from build123d import *

# Parameters (mm, degrees)
ESBO_O1_W                = 113
ESBO_O1_H                = 26.5
RESSALTO_EXTRUS_O1_DEPTH = 5
ESBO_O2_W                = 5
ESBO_O2_H                = 7.62
CORTE_EXTRUS_O1_DEPTH    = 5
CORTE_EXTRUS_O2_DEPTH    = 5
ESBO_O4_R                = 1.6
CORTE_EXTRUS_O3_DEPTH    = 10


with BuildPart() as part:
    # Esboço1 → Ressalto-extrusão1 (new body)
    with BuildSketch(Plane(origin=(0, 0, 0), x_dir=(1, 0, 0), z_dir=(0, 1, 0))):
        with Locations((-20.23644711, -18.909257917)):
            Rectangle(ESBO_O1_W, ESBO_O1_H)
    extrude(amount=RESSALTO_EXTRUS_O1_DEPTH)

    # Esboço2 → Corte-extrusão1 (cut)
    with BuildSketch(Plane(origin=(0, 5, 0), x_dir=(1, 0, 0), z_dir=(0, 1, 0))):
        with Locations((13.76355289, -18.914257917)):
            Rectangle(ESBO_O2_W, ESBO_O2_H)
        with Locations((-54.23644711, -18.914257917)):
            Rectangle(ESBO_O2_W, ESBO_O2_H)
    extrude(amount=-CORTE_EXTRUS_O1_DEPTH, mode=Mode.SUBTRACT)

    # Esboço3 → Corte-extrusão2 (cut)
    with BuildSketch(Plane(origin=(0, 5, 0), x_dir=(1, 0, 0), z_dir=(0, 1, 0))):
        Polygon((-76.73644711, -17.909257917), (-73.23644711, -17.909257917), (-73.23644711, -16.109257917), (-71.73644711, -16.109257917), (-71.73644711, -17.909257917), (-69.73644711, -17.909257917), (-69.73644711, -19.909257917), (-71.73644711, -19.909257917), (-71.73644711, -21.709257917), (-73.23644711, -21.709257917), (-73.23644711, -19.909257917), (-76.73644711, -19.909257917), align=None)
        Polygon((-51.73644711, -17.909257917), (-48.23644711, -17.909257917), (-48.23644711, -16.109257917), (-46.73644711, -16.109257917), (-46.73644711, -17.909257917), (-44.73644711, -17.909257917), (-44.73644711, -19.909257917), (-46.73644711, -19.909257917), (-46.73644711, -21.709257917), (-48.23644711, -21.709257917), (-48.23644711, -19.909257917), (-51.73644711, -19.909257917), align=None)
    corte_extrus_o2 = extrude(amount=-CORTE_EXTRUS_O2_DEPTH, mode=Mode.SUBTRACT)

    # Espelhar1: Corte-extrusão2 across plane
    add(corte_extrus_o2.mirror(Plane.ZY.offset(20.23644711)), mode=Mode.SUBTRACT)

    # Esboço4 → Corte-extrusão3 (cut)
    with BuildSketch(Plane(origin=(0, 0, 0), x_dir=(-1, 0, 0), z_dir=(0, -1, 0))):
        with Locations(Location((1.56644711, -10.659257917, 0), (0, 0, 90))):
            Circle(ESBO_O4_R)
        with Locations(Location((38.90644711, -10.659257917, 0), (0, 0, 90))):
            Circle(ESBO_O4_R)
    extrude(amount=-CORTE_EXTRUS_O3_DEPTH, mode=Mode.SUBTRACT)


solid = part.part
Part model, mm, in its own coordinate system. A direction names the side the tool comes from. Coordinates: 2 decimals unless noted, no trailing zeros. Loops run counter-clockwise (first coordinate to the right, second up) from the corner with the lowest first, then second, coordinate; pieces in that order, holes last. Notation, with made-up numbers: (43, 62.5) - (88, 62.5) arc R35 ccw to (88, 97.5) - close; hole circle Ø10 at (75, -30). An arc over 180 degrees is marked (long way). Write each question's results on one line, items separated by ' | '. Start each with the question number.
Q1. Which spindle directions (+Z, -Z, +X, -X, +Y, -Y) get a long thin tool onto all of the face, cutting with end or side? Do faces 1 (the flat face through (-75, 3, 17.909)), 2 (the flat face through (34, 3, 19.909)), 3 (the flat face through (-51.736, 3, 17)). Say none if no direction does.
Q2. Two-plate mould, pull along Z, no slides. Class faces 4 (the flat face through (-76.736, 2, 26)), 5 (the flat face through (31.264, 3, 17)): +Z half, -Z half, draft (parallel to the pull), parting line (faces both ways), or undercut.
Q3. Drop a flat-ended pin along its axis: pin 1 Ø1.9 at (x, z) = (-38.91, 10.66) entering from +Y. Give the stop position or say it passes through.
Q4. Probe line 1 along X through (y, z) = (3.5, 18); line 2 along Z through (x, y) = (13.5, 2.8); line 3 along Z through (x, y) = (-48, 3.45). List the from-to ranges inside material, lowest first.
Q5. Slice it at A-A on x = 13. Give the cut face in (y, z).
Q6. Slice it at B-B on y = 3.55. Give the number of separate pieces and of enclosed holes in the cut face, and give its area (3 significant figures).
Answer:
1) face 1: -X, +Y, -Y | face 2: +X, +Y, -Y | face 3: +Y, -Y
2) face 4: draft | face 5: undercut
3) pin 1: passes through
4) line 1: x = -69.74 to -56.74, -44.74 to 4.26, 16.26 to 29.26 | line 2: z = 5.66 to 15.1, 22.72 to 32.16 | line 3: z = 5.66 to 16.11, 21.71 to 32.16
5) outline: (0, 5.66) - (5, 5.66) - (5, 15.1) - (0, 15.1) - close; (0, 22.72) - (5, 22.72) - (5, 32.16) - (0, 32.16) - close
6) separate pieces: 1 | enclosed holes: 4 | area: 2,820 mm2
